from build123d import *

# Parameters (mm, degrees)
SKETCH3_R           = 0.775
BOSS_EXTRUDE1_DEPTH = 2.25


with BuildPart() as part:
    # Sweep1: sweep along a path in Sketch1
    with BuildLine(Plane(origin=(0, 0, 0), x_dir=(0, 0, -1), z_dir=(1, 0, 0))) as sweep1_path:
        CenterArc((0, 0), 4.15, 0, 360)
    # Sketch2 → Sweep1 (sweep)
    with BuildSketch(Plane.XY):
        with BuildLine():
            Line((6.75, 0), (-6.75, 0))
            Line((-6.75, 0), (-6.75, 3.32420652))
            ThreePointArc((-6.75, 3.32420652), (0, 4.15), (6.75, 3.32420652))
            Line((6.75, 3.32420652), (6.75, 0))
        make_face()
    sweep(path=sweep1_path.line)

    # Sketch3 → Boss-Extrude1 (add)
    with BuildSketch(Plane.ZY.offset(6.75)):
        Circle(SKETCH3_R)
    boss_extrude1 = extrude(amount=BOSS_EXTRUDE1_DEPTH)

    # Mirror1: Boss-Extrude1 across plane
    add(boss_extrude1.mirror(Plane(origin=(0, 0, 0), x_dir=(0, 0, 1), z_dir=(1, 0, 0))))


solid = part.part
The model under review builds one solid part; all positions refer to its coordinate system, in mm. A direction names the side the tool comes from. Give positions to 0.01 mm unless a question says otherwise; leave off trailing zeros. Answer in a Markdown table with one row per item. Add a question column.
1. To check wall thickness, follow line 1 along X through (y, z) = (0, 1.5); line 2 along Z through (x, y) = (-5.5, 3); line 3 along Y through (x, z) = (1.75, -1). State the ranges of each line that lie inside material, in increasing order.
2. For pin 1 Ø3 at (x, z) = (6.5, 0) entering from +Y; pin 2 Ø1 at (x, y) = (-6, -2.5) entering from +Z; pin 3 Ø4 at (y, z) = (0.5, -3) entering from -X, all flat-tipped, find the tip position at first contact; note any pin that passes through.
3. Machinability: for faces 1 (the flat face through (9, 0, 0)), 2 (the cylindrical face through (-7.859, -0.688, 0.358)), 3 (the cylindrical face through (7.859, -0.688, 0.358)), which of the approach directions +Z, -Z, +X, -X, +Y, -Y give a long, thin tool a straight path to every point of the face, cutting with its end or side? Answer none if there is none.
The answers:
| question | item | result |
|---|---|---|
| 1 | line 1 | -6.75 to 6.75 |
| 1 | line 2 | -2 to 2 |
| 1 | line 3 | -3.97 to 3.97 |
| 2 | pin 1 | y = 3.7 |
| 2 | pin 2 | z = 2.9 |
| 2 | pin 3 | x = -6.75 |
| 3 | face 1 | +Z, -Z, +X, +Y, -Y |
| 3 | face 2 | -X |
| 3 | face 3 | +X |
